Geometry check sheet. Reference: drawing and pictorial views, mm from the part's lowest x, y, z. A direction names the side the tool comes from. Give positions to 0.01 mm unless a question says otherwise; leave off trailing zeros. Order: outer loops, then holes, each group sorted by start corner. A loop starts at its lowest first (then second) coordinate and runs counter-clockwise, first axis right, second up.
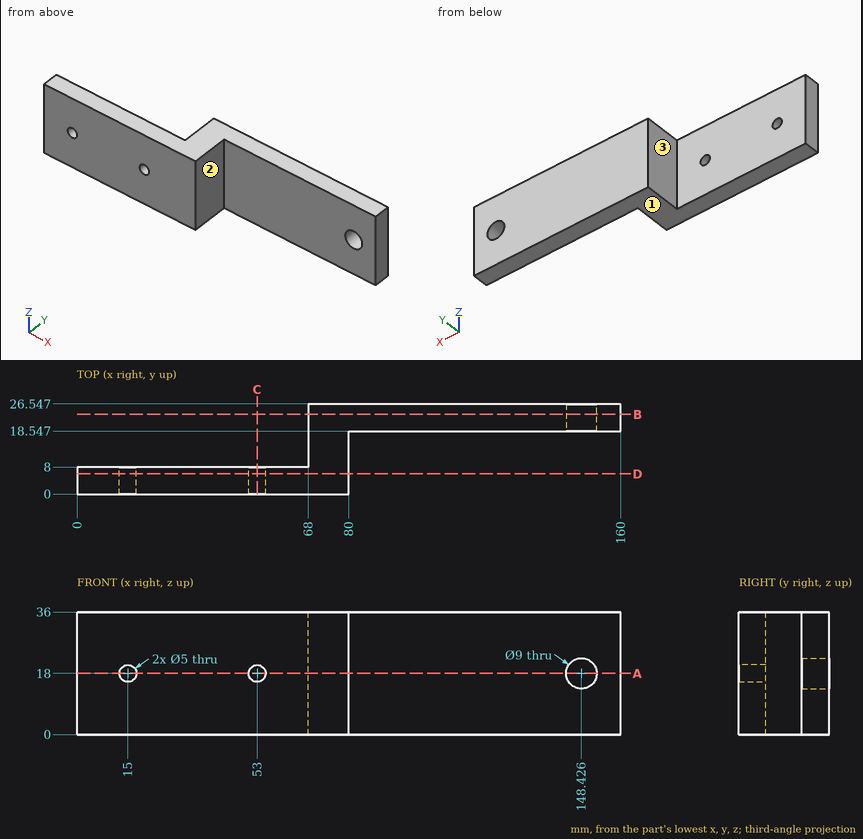
(1) Cross-section at B-B on y = 23.5. Enter the section's corners in (x, z), then the cut area to 3 significant figures.
Response values:
outline: (68, 0) - (160, 0) - (160, 36) - (68, 36) - close; hole circle Ø9 at (148.43, 18)
area: 3,250 mm2
(2) Cross-section at C-C on x = 53. Enter the section's corners in (y, z).
Response values:
outline: (0, 0) - (8, 0) - (8, 15.5) - (0, 15.5) - close; (0, 20.5) - (8, 20.5) - (8, 36) - (0, 36) - close
(3) Cross-section at D-D on y = 6. Enter the section's corners in (x, z).
Response values:
outline: (0, 0) - (80, 0) - (80, 36) - (0, 36) - close; hole circle Ø5 at (15, 18); hole circle Ø5 at (53, 18)
(4) Gauge pin test, flat ends, axial feed: pin 1 Ø4.5 at (x, z) = (15, 18) entering from -Y; pin 2 Ø8 at (x, z) = (104.5, 11) entering from -Y; pin 3 Ø3 at (y, z) = (22, 16.5) entering from -X. Record the tip position at first contact, or that the pin passes through.
Response values:
pin 1: passes through
pin 2: stops at y = 18.55
pin 3: stops at x = 68
(5) Cross-section at A-A on z = 18. Enter the section's corners in (x, y).
Response values:
outline: (0, 0) - (12.5, 0) - (12.5, 8) - (0, 8) - close; (17.5, 0) - (50.5, 0) - (50.5, 8) - (17.5, 8) - close; (55.5, 0) - (80, 0) - (80, 18.55) - (143.93, 18.55) - (143.93, 26.55) - (68, 26.55) - (68, 8) - (55.5, 8) - close; (152.93, 18.55) - (160, 18.55) - (160, 26.55) - (152.93, 26.55) - close
(6) Material ranges on L1, parallel to X at y = 3.5, z = 18; L2, parallel to Y at x = 56, z = 26; L3, parallel to Y at x = 149.5, z = 23.5, recorded low to high.
Response values:
L1: x = 0 to 12.5, 17.5 to 50.5, 55.5 to 80
L2: y = 0 to 8
L3: y = 18.55 to 26.55
(7) Set-up check for the marked faces 1, 2 and 3: record each of +Z, -Z, +X, -X, +Y, -Y from which the full face is reachable in a straight line by a thin tool's end or side.
Response values:
face 1: -Z, +X, -X, +Y, -Y
face 2: +Z, -Z, +X, -Y
face 3: +Z, -Z, -X, +Y
